```python
from build123d import *

# Parameters (mm, degrees)
F0_W     = 100
F0_H     = 50
F1_DEPTH = 50
F3_DEPTH = 40
F4_R     = 40
F5_SIZE  = 5
F6_SIZE  = 5
F7_SIZE  = 5


with BuildPart() as f1:
    # F0 (on Front) → F1 (new body, symmetric)
    with BuildSketch(Plane.XZ):
        with Locations((-0.236801, -24.486255)):
            Rectangle(F0_W, F0_H)
    extrude(amount=F1_DEPTH, both=True)

    # F2 (on Right) → F3 (cut, symmetric)
    with BuildSketch(Plane.YZ):
        Polygon((20.232478, -35.412774), (40, 10.513745), (0, 10.513745), (-19.767522, -35.412774), align=None)
    extrude(amount=F3_DEPTH, both=True, mode=Mode.SUBTRACT)

    # F4
    f4_edges = [f1.edges().sort_by_distance(p)[0] for p in [
        (-0.236801, -50, 0.513745),
    ]]
    fillet(f4_edges, radius=F4_R)

    # F5
    f5_edges = [f1.edges().sort_by_distance(p)[0] for p in [
        (-50.236801, 20, 0.513745),
    ]]
    chamfer(f5_edges, length=F5_SIZE)

    # F6
    f6_edges = [f1.edges().sort_by_distance(p)[0] for p in [
        (49.763199, 20, 0.513745),
    ]]
    chamfer(f6_edges, length=F6_SIZE)

    # F7
    f7_edges = [f1.edges().sort_by_distance(p)[0] for p in [
        (-0.236801, 50, 0.513745),
    ]]
    chamfer(f7_edges, length=F7_SIZE)


solid = f1.part
```
Geometry: final body of the model. Coordinates: model frame, mm. A direction names the side the tool comes from. Round coordinates to 2 decimals unless told otherwise and drop trailing zeros. Write each loop counter-clockwise with the first axis right and the second up, starting at its lowest first coordinate (ties: lowest second). Pieces come first, ordered by that corner, then holes. Notation, with made-up numbers: M -2,24 L 56,24 A16 ccw 56,43 Z; hole C 38,63 d2. An arc over 180 degrees is marked long. Answer in a Markdown table with one row per item. Add a question column.
(1) Cut plane A-A, the plane y = 14. Return the cut outline in (x, z), then the cut area to 3 significant figures.
(2) Ray query, L1, parallel to X at y = 6, z = -29; L2, parallel to Z at x = 8, y = 6; L3, parallel to X at y = 16.5, z = -2. Return the intervals inside material, ascending.
(3) Cut plane B-B, the plane x = 28. Return the cut outline in (y, z).
(4) Reachability of faces 1 (the face through (-40, 8, -17)), 2 (the face through (0.56, 27.856, -17.701)), 3 (the face through (-1, -1, -49.486)) from +Z, -Z, +X, -X, +Y, -Y: full face, straight path, thin tool, end or side. Return the list, or none.
(5) Draft query along Z for faces 4 (the face through (40, 8, -17)), 5 (the face through (0.56, -11.93, -17.2)), 6 (the face through (47.298, -47.465, -44.556)), 7 (the face through (-49.368, -35.64, -14.404)). Return one class per face: pulls with the +Z half, pulls with the -Z half, needs draft (parallel to the pull), parting line crosses it, or undercut.
(6) Contact query for flat-ended pins moving along their axis: pin 1 (3 mm diameter, centred on x = -1, z = -18, fed in from -Y); pin 2 (1.5 mm diameter, centred on x = 27, z = -13.5, fed in from -Y). Output: stop coordinate, or through.
Established:
| question | item | result |
|---|---|---|
| 1 | outline | M -50.24,-49.49 L 49.76,-49.49 L 49.76,-4.49 L 44.76,0.51 L 40,0.51 L 40,-35.41 L -40,-35.41 L -40,0.51 L -45.24,0.51 L -50.24,-4.49 Z |
| 1 | area | 2,100 mm² |
| 2 | L1 | -50.24 to -40, 40 to 49.76 |
| 2 | L2 | -49.49 to -35.41 |
| 2 | L3 | -47.75 to -40, 40 to 47.28 |
| 3 | outline | M -50,-49.49 L 50,-49.49 L 50,-4.49 L 45,0.51 L 35.7,0.51 L 20.23,-35.41 L -19.77,-35.41 L -4.3,0.51 L -10,0.51 A40 ccw -50,-39.49 Z |
| 4 | face 1 | none |
| 4 | face 2 | +Z |
| 4 | face 3 | -Z, +X, -X, +Y, -Y |
| 5 | face 4 | undercut |
| 5 | face 5 | undercut |
| 5 | face 6 | needs draft |
| 5 | face 7 | pulls with the +Z half |
| 6 | pin 1 | y = -44.65 |
| 6 | pin 2 | y = -41.03 |
